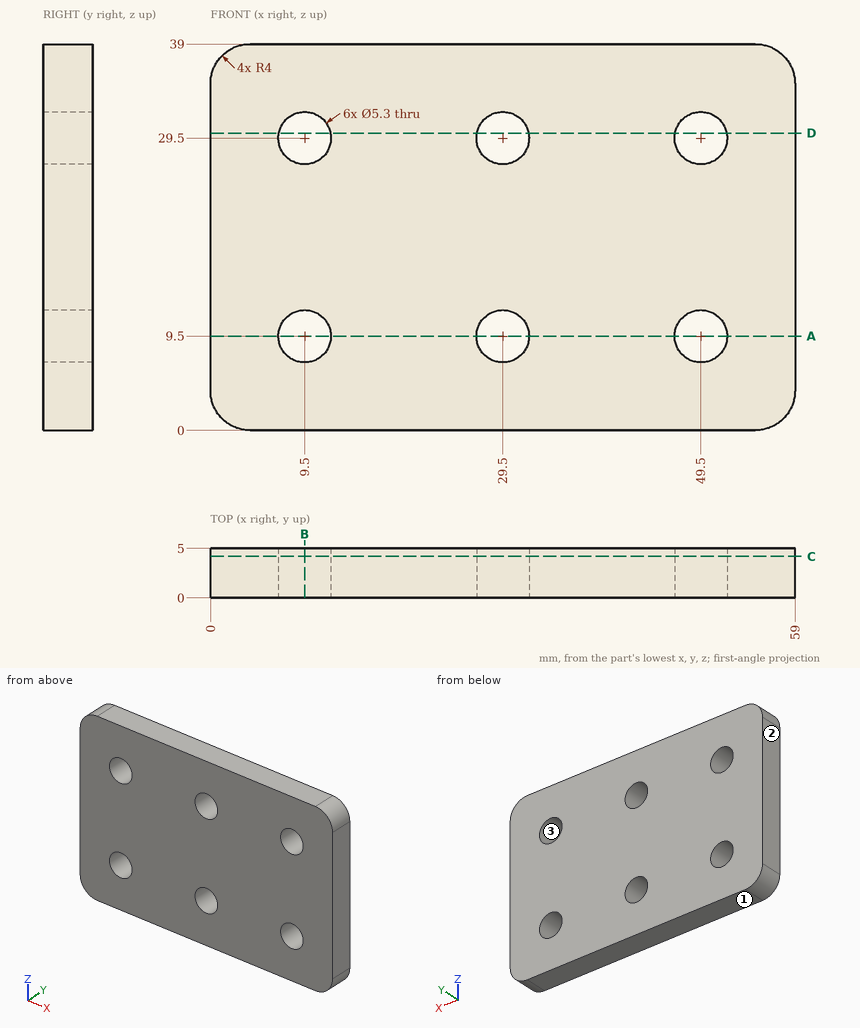
For this review, use the dimensioned drawing (mm, ordinates from the lowest corner) and the shaded views. Coordinates: 2 decimals unless noted, no trailing zeros. Loops run counter-clockwise (first coordinate to the right, second up) from the corner with the lowest first, then second, coordinate; pieces in that order, holes last. Notation, with made-up numbers: (81.5, -37.5) - (87.5, -37.5) arc R29 cw to (87.5, -6.5) - close; hole circle Ø6 at (-4.5, 88). An arc over 180 degrees is marked (long way). Use CSV: the item, a comma, the result in double quotes. Start each with the question number.
1) Consider section B-B on x = 9.5. Write out the cut boundary in (y, z), then the cut area to 3 significant figures.
2) Consider section D-D on z = 30. Write out the cut boundary in (x, y).
3) Consider section C-C on y = 4.2. Write out the cut boundary in (x, z), then the cut area to 3 significant figures.
4) Wall thickness on L1, parallel to X at y = 1.8, z = 29.5; L2, parallel to Z at x = 11.5, y = 4.4; L3, parallel to X at y = 1.85, z = 28: over which ranges is each line inside the solid? List them lowest first. Write a range as from..to.
5) The part is to be moulded in two halves that separate along Z. For the marked faces 1, 2 and 3, say which applies: +Z half, -Z half, draft (parallel to the pull), parting line (faces both ways), or undercut.
6) Consider section A-A on z = 9.5. Write out the cut boundary in (x, y), then the cut area to 4 significant figures.
Geometry says:
1,outline,"(0, 0) - (5, 0) - (5, 6.85) - (0, 6.85) - close; (0, 12.15) - (5, 12.15) - (5, 26.85) - (0, 26.85) - close; (0, 32.15) - (5, 32.15) - (5, 39) - (0, 39) - close"
1,area,"142 mm^2"
2,outline,"(0, 0) - (6.9, 0) - (6.9, 5) - (0, 5) - close; (12.1, 0) - (26.9, 0) - (26.9, 5) - (12.1, 5) - close; (32.1, 0) - (46.9, 0) - (46.9, 5) - (32.1, 5) - close; (52.1, 0) - (59, 0) - (59, 5) - (52.1, 5) - close"
3,outline,"(0, 4) arc R4 ccw to (4, 0) - (55, 0) arc R4 ccw to (59, 4) - (59, 35) arc R4 ccw to (55, 39) - (4, 39) arc R4 ccw to (0, 35) - close; hole circle Ø5.3 at (9.5, 9.5); hole circle Ø5.3 at (9.5, 29.5); hole circle Ø5.3 at (29.5, 9.5); hole circle Ø5.3 at (29.5, 29.5); hole circle Ø5.3 at (49.5, 9.5); hole circle Ø5.3 at (49.5, 29.5)"
3,area,"2,150 mm^2"
4,L1,"0..6.85, 12.15..26.85, 32.15..46.85, 52.15..59"
4,L2,"0..7.76, 11.24..27.76, 31.24..39"
4,L3,"0..7.32, 11.68..27.32, 31.68..47.32, 51.68..59"
5,face 1,"-Z half"
5,face 2,"draft"
5,face 3,"undercut"
6,outline,"(0, 0) - (6.85, 0) - (6.85, 5) - (0, 5) - close; (12.15, 0) - (26.85, 0) - (26.85, 5) - (12.15, 5) - close; (32.15, 0) - (46.85, 0) - (46.85, 5) - (32.15, 5) - close; (52.15, 0) - (59, 0) - (59, 5) - (52.15, 5) - close"
6,area,"215.5 mm^2"
